Design review of the part built by this model. Coordinates are the model's own, in mm. A direction names the side the tool comes from. Coordinates: 2 decimals unless noted, no trailing zeros. Write each loop counter-clockwise with the first axis right and the second up, starting at its lowest first coordinate (ties: lowest second). Pieces come first, ordered by that corner, then holes. Notation, with made-up numbers: (74.25, -23.75) - (82.25, -23.75) arc R18 ccw to (82.25, 4.25) - close; hole circle Ø4 at (9.5, -23.75). An arc over 180 degrees is marked (long way). Use a Markdown table: item, result.
Autodesk Inventor part; units mm, degrees
ref_plane "YZ Plane" through (0, 0, 0) normal (1, 0, 0) x (0, 1, 0)
ref_plane "XZ Plane" through (0, 0, 0) normal (0, 1, 0) x (-1, 0, 0)
ref_plane "XY Plane" through (0, 0, 0) normal (0, 0, 1) x (1, 0, 0)
sketch "Sketch2" plane through (0, 0, 0) normal (0, 0, 1) x (1, 0, 0)
  circle A0 centre (0, 0) radius 4
  dimension "d0" = 8
extrude "Extrusion1" add sketch "Sketch2" against normal blind 20
sketch "Sketch3" plane through (0, 0, 0) normal (0, 0, 1) x (1, 0, 0)
  circle A0 centre (0, 0) radius 4
  line L0 (-4, 3) -> (4, 3)
  line L1 (4, 3) -> (4, -3)
  line L2 (4, -3) -> (-4, -3)
  line L3 (-4, -3) -> (-4, 3)
  line L4 (-4, 3) -> (4, 3)
  line L5 (4, 3) -> (4, 4)
  line L6 (4, 4) -> (-4, 4)
  line L7 (-4, 4) -> (-4, 3)
  line L8 (-4, 0) -> (4, 0) construction
  point P0 (4, 3.5)
  dimension "d3" = 6
extrude "Extrusion2" cut sketch "Sketch3" against normal up to surface (20 mm away) from surface at 0 contours L0 A0 | A0 L6 L5 L0 | A0 L0 L7 L6
mirror "Mirror1" about plane through (0, 0, 0) normal (0, 1, 0) of "Extrusion2"
sketch "Sketch5" plane through (0, 0, 0) normal (0, 0, 1) x (1, 0, 0)
  circle A0 centre (0, 0) radius 1.75
  dimension "d6" = 3.5
extrude "Extrusion3" add sketch "Sketch5" along normal blind 0.5
sketch "Sketch6" plane through (0, 0, 0) normal (0, 0, 1) x (1, 0, 0)
  circle A0 centre (0, 0) radius 0.5
  dimension "d9" = 1
extrude "Extrusion4" add sketch "Sketch6" along normal blind 8
sketch "Sketch7" plane through (0, 0, 8) normal (0, 0, 1) x (1, 0, 0)
  circle A0 centre (0, 0) radius 5.25
  dimension "d12" = 10.5
extrude "Extrusion5" add sketch "Sketch7" against normal blind 5
sketch "Sketch8" plane through (0, 0, 8) normal (0, 0, 1) x (1, 0, 0)
  circle A0 centre (0, 0) radius 5.25
  line L0 (-2, 1.5) -> (2, 1.5)
  line L1 (2, 1.5) -> (2, 0)
  line L2 (2, 0) -> (-2, 0)
  line L3 (-2, 0) -> (-2, 1.5)
  line L4 (-5.25, 0) -> (5.25, 0)
  dimension "d15" = 4
  dimension "d16" = 1.5
extrude "Extrusion6" cut sketch "Sketch8" against normal up to surface (5 mm away) contours L4 L1 L0 L3 A0
sketch "Sketch9" plane through (0, 0, -20) normal (0, 0, -1) x (-1, 0, 0)
  circle A0 centre (0, 0) radius 1.75
  dimension "d19" = 3.5
extrude "Extrusion7" add sketch "Sketch9" along normal blind 1
sketch "Sketch10" plane through (0, 0, -20) normal (0, 0, -1) x (-1, 0, 0)
  circle A0 centre (0, 0) radius 1.75
  line L0 (-2.6458, -3) -> (2.6458, -3)
  arc A1 (2.6458, -3) -> (2.6458, 3) centre (0, 0) ccw
  line L1 (2.6458, 3) -> (-2.6458, 3)
  arc A2 (-2.6458, 3) -> (-2.6458, -3) centre (0, 0) ccw
  arc A3 (-2.6458, 3) -> (-2.6458, -3) centre (0, 0) ccw construction
  line L2 (-4, 0) -> (4, 0) construction
  arc A4 (2.6458, -3) -> (2.6458, 3) centre (0, 0) ccw construction
  line L3 (-3.9392, 0.6946) -> (3.9392, -0.6946) construction
  line L4 (-3.0153, 1.0394) -> (-2.7199, 0.9873)
  line L5 (-2.7199, 0.9873) -> (-2.8935, 0.0025)
  line L6 (-2.8935, 0.0025) -> (-3.189, 0.0546)
  line L7 (-3.189, 0.0546) -> (-3.0153, 1.0394)
  line L8 (0.3039, 1.7234) -> (-0.3039, -1.7234) construction
  line L9 (3.189, -0.0546) -> (2.8935, -0.0025)
  line L10 (2.8935, -0.0025) -> (2.7199, -0.9873)
  line L11 (2.7199, -0.9873) -> (3.0153, -1.0394)
  line L12 (3.0153, -1.0394) -> (3.189, -0.0546)
  point P0 (0, 0)
  dimension "d22" = 10
  dimension "d23" = 0.3
  dimension "d24" = 1
  dimension "d25" = 0.5
  dimension "d26" = 2.85
extrude "Extrusion8" add sketch "Sketch10" along normal blind 1 contours L4 L5 L6 L7 | L12 L11 L10 L9
ref_plane "Work Plane1" through (0, 0, 0) normal (0, 1, 0) x (-1, 0, 0)
equation "\"d25\" = 0.5 * d24"
properties part number "308-106"
(1) Draft analysis for pull direction Z (two halves, no side actions). For faces 1 (the cylindrical face through (-4, 0, -10)), 2 (the cylindrical face through (1.617, 0.67, 0.246)), 3 (the flat face through (-2, 0, -20)), 4 (the flat face through (0, -2, 3)), state which applies: +Z half, -Z half, draft (parallel to the pull), parting line (faces both ways), or undercut.
Determined:
| item | result |
|---|---|
| face 1 | draft |
| face 2 | undercut |
| face 3 | -Z half |
| face 4 | undercut |
(2) For pin 1 (1.6 mm diameter, centred on x = -1.5, z = -6.5, fed in from -Y); pin 2 (3 mm diameter, centred on y = 2, z = -5.5, fed in from -X); pin 3 (1.5 mm diameter, centred on y = -4.5, z = 2.5, fed in from -X); pin 4 (1.5 mm diameter, centred on x = -3.5, y = 0, fed in from -Z), all flat-tipped, find the tip position at first contact; note any pin that passes through.
Determined:
| item | result |
|---|---|
| pin 1 | y = -3 |
| pin 2 | x = -3.97 |
| pin 3 | x = -3.47 |
| pin 4 | z = -21 |
(3) For L1, parallel to Z at x = -0.75, y = -0.5; L2, parallel to Z at x = 2, y = -2.5; L3, parallel to Z at x = 1.5, y = 1.75, list the stretches that pass through material, from the lowest coordinate up. Write a range as from..to.
Determined:
| item | result |
|---|---|
| L1 | -21..0.5, 3..8 |
| L2 | -20..0, 3..8 |
| L3 | -20..0 |
(4) Take a section at C-C on z = -3.5. Write out the cut boundary in (x, y).
Determined:
| item | result |
|---|---|
| outline | (-2.65, -3) - (2.65, -3) arc R4 ccw to (2.65, 3) - (-2.65, 3) arc R4 ccw to start |
(5) Take a section at A-A on x = 0. Write out the cut boundary in (y, z).
Determined:
| item | result |
|---|---|
| outline | (-5.25, 3) - (-0.5, 3) - (-0.5, 0.5) - (-1.75, 0.5) - (-1.75, 0) - (-3, 0) - (-3, -20) - (-1.75, -20) - (-1.75, -21) - (1.75, -21) - (1.75, -20) - (3, -20) - (3, 0) - (1.75, 0) - (1.75, 0.5) - (0.5, 0.5) - (0.5, 3) - (1.5, 3) - (1.5, 8) - (-5.25, 8) - close |
(6) Machinability: for faces 5 (the flat face through (2.805, 0.502, -20.493)), 6 (the flat face through (4, 0, 6)), 7 (the flat face through (0, 1.5, 6)), which of the approach directions +Z, -Z, +X, -X, +Y, -Y give a long, thin tool a straight path to every point of the face, cutting with its end or side? Answer none if there is none.
Determined:
| item | result |
|---|---|
| face 5 | -Z, -Y |
| face 6 | +Z, +X, +Y |
| face 7 | +Z, +X, -X, +Y |
(7) Take a section at B-B on z = 6.25. Write out the cut boundary in (x, y), and give its area (3 significant figures).
Determined:
| item | result |
|---|---|
| outline | (-5.25, 0) arc R5.25 ccw to (5.25, 0) - (2, 0) - (2, 1.5) - (-2, 1.5) - (-2, 0) - close |
| area | 49.3 mm2 |
